For this review, take the finished solid that the model builds, in its own axes (mm). A direction names the side the tool comes from. Coordinates: 2 decimals unless noted, no trailing zeros. Loops run counter-clockwise (first coordinate to the right, second up) from the corner with the lowest first, then second, coordinate; pieces in that order, holes last. Notation, with made-up numbers: M 5.5,-11 L 10.5,-11 A15 ccw 10.5,-5 Z; hole C 89,80 d9. An arc over 180 degrees is marked long. Use one line per item in the form item = value.
```python
from build123d import *

# Parameters (mm, degrees)
SKETCH1_W           = 47
SKETCH1_H           = 55.5
BOSS_EXTRUDE1_DEPTH = 15
CUT_EXTRUDE4_DEPTH  = 54
FILLET1_R           = 7
FILLET2_R           = 7
SKETCH3_W           = 4.401923789
SKETCH3_H           = 6.5
CUT_EXTRUDE5_DEPTH  = 54
SKETCH4_W           = 1
SKETCH4_H           = 1
CUT_EXTRUDE6_DEPTH  = 54
CUT_EXTRUDE7_DEPTH  = 20
CUT_EXTRUDE8_DEPTH  = 5
BOSS_EXTRUDE3_DEPTH = 1.5
CUT_EXTRUDE9_DEPTH  = 57


with BuildPart() as part:
    # Sketch1 → Boss-Extrude1 (new body)
    with BuildSketch(Plane(origin=(0, 0, 0), x_dir=(1, 0, 0), z_dir=(0, 1, 0))):
        with Locations((23.5, -27.75)):
            Rectangle(SKETCH1_W, SKETCH1_H)
    extrude(amount=BOSS_EXTRUDE1_DEPTH)

    # Sketch2 → Cut-Extrude4 (cut)
    with BuildSketch(Plane.XY.offset(55.5)):
        with BuildLine():
            ThreePointArc((11.098076211, 15), (8.5, 15.5), (5.901923789, 15))
            Line((5.901923789, 15), (11.098076211, 15))
        make_face()
        with BuildLine():
            Line((11.098076211, 15), (5.901923789, 15))
            ThreePointArc((5.901923789, 15), (4.574858823, 2.70403013), (15.5, 8.5))
            ThreePointArc((15.5, 8.5), (14.29596987, 12.425141177), (11.098076211, 15))
        make_face()
        with BuildLine():
            ThreePointArc((26.098076211, 15), (23.5, 15.5), (20.901923789, 15))
            Line((20.901923789, 15), (26.098076211, 15))
        make_face()
        with BuildLine():
            Line((26.098076211, 15), (20.901923789, 15))
            ThreePointArc((20.901923789, 15), (19.574858823, 2.70403013), (30.5, 8.5))
            ThreePointArc((30.5, 8.5), (29.29596987, 12.425141177), (26.098076211, 15))
        make_face()
        with BuildLine():
            ThreePointArc((45.5, 8.5), (44.29596987, 12.425141177), (41.098076211, 15))
            Line((41.098076211, 15), (35.901923789, 15))
            ThreePointArc((35.901923789, 15), (34.574858823, 2.70403013), (45.5, 8.5))
        make_face()
        with BuildLine():
            Line((35.901923789, 15), (41.098076211, 15))
            ThreePointArc((41.098076211, 15), (38.5, 15.5), (35.901923789, 15))
        make_face()
    extrude(amount=-CUT_EXTRUDE4_DEPTH, mode=Mode.SUBTRACT)

    # Fillet1
    fillet1_edges = [part.edges().sort_by_distance(p)[0] for p in [
        (47, 15, 27.75),
    ]]
    fillet(fillet1_edges, radius=FILLET1_R)

    # Fillet2
    fillet2_edges = [part.edges().sort_by_distance(p)[0] for p in [
        (0, 15, 27.75),
    ]]
    fillet(fillet2_edges, radius=FILLET2_R)

    # Sketch3 → Cut-Extrude5 (cut)
    with BuildSketch(Plane.XY.offset(55.5)):
        with Locations((28.299038106, 11.75)):
            Rectangle(SKETCH3_W, SKETCH3_H)
        with Locations((33.700961895, 11.75)):
            Rectangle(SKETCH3_W, SKETCH3_H)
        with Locations((13.299038106, 11.75)):
            Rectangle(SKETCH3_W, SKETCH3_H)
        with Locations((18.700961895, 11.75)):
            Rectangle(SKETCH3_W, SKETCH3_H)
    extrude(amount=-CUT_EXTRUDE5_DEPTH, mode=Mode.SUBTRACT)

    # Sketch4 → Cut-Extrude6 (cut)
    with BuildSketch(Plane.XY.offset(55.5)):
        with Locations((16, 14.5)):
            Rectangle(SKETCH4_W, SKETCH4_H)
        with Locations((31, 14.5)):
            Rectangle(SKETCH4_W, SKETCH4_H)
    extrude(amount=-CUT_EXTRUDE6_DEPTH, mode=Mode.SUBTRACT)

    # Sketch5 → Cut-Extrude7 (cut)
    with BuildSketch(Plane.ZY.offset(-15.5)):
        Polygon((6.5, 14), (50.5, 14), (40.5, 7), (16.5, 7), align=None)
    extrude(amount=-CUT_EXTRUDE7_DEPTH, mode=Mode.SUBTRACT)

    # Sketch5_2 → Cut-Extrude8 (cut)
    with BuildSketch(Plane.ZY.offset(-15.5)):
        Polygon((6.5, 14), (50.5, 14), (40.5, 7), (16.5, 7), align=None)
    extrude(amount=CUT_EXTRUDE8_DEPTH, mode=Mode.SUBTRACT)

    # Sketch6 → Boss-Extrude3 (add)
    with BuildSketch(Plane.XY.offset(55.5)):
        with BuildLine():
            Line((0, 0), (47, 0))
            Line((47, 0), (47, 8))
            ThreePointArc((47, 8), (44.949747468, 12.949747468), (40, 15))
            Line((40, 15), (7, 15))
            ThreePointArc((7, 15), (2.050252532, 12.949747468), (0, 8))
            Line((0, 8), (0, 0))
        make_face()
    extrude(amount=BOSS_EXTRUDE3_DEPTH)

    # Sketch7 → Cut-Extrude9 (cut)
    with BuildSketch(Plane.XY.offset(57)):
        Polygon((16, 8), (16, 15), (47, 15), (47, 0), (16, 0), align=None)
    extrude(amount=-CUT_EXTRUDE9_DEPTH, mode=Mode.SUBTRACT)

    # Mirror1: part across plane


with BuildPart() as part_1:
    add(part.part)
    add(part.part.mirror(Plane(origin=(16, 8, 0), x_dir=(0, 0, 1), z_dir=(-1, 0, 0))))


solid = part_1.part
```
1. Consider section B-B on y = 12.25. Write out the cut boundary in (x, z).
Computed values:
outline = M 1.44,0 L 30.56,0 L 30.56,57 L 1.44,57 Z; hole M 2.59,1.5 L 15.5,1.5 L 15.5,9 L 16.5,9 L 16.5,1.5 L 29.41,1.5 L 29.41,55.5 L 16.5,55.5 L 16.5,48 L 15.5,48 L 15.5,55.5 L 2.59,55.5 Z
2. Tool access review of faces 4 (the face through (16, 15, 1)), 5 (the face through (27.44, 2.714, 28.878)), 6 (the face through (15.5, 11, 51)): name each direction out of +Z, -Z, +X, -X, +Y, -Y from which nothing blocks a thin tool from reaching the whole face with its end or side.
Computed values:
face_4 = +Z, -Z, +X, -X, +Y
face_5 = none
face_6 = +Y
3. Consider section C-C on z = 46. Write out the cut boundary in (x, y).
Computed values:
outline = M 0,0 L 32,0 L 32,8 A7 ccw 26.45,14.85 A7 cw long 16.5,8.5 L 16.5,10.85 L 15.5,10.85 L 15.5,8.5 A7 cw long 5.55,14.85 A7 ccw 0,8 Z
4. Consider section A-A on x = 8.5. Write out the cut boundary in (y, z).
Computed values:
outline = M 0,0 L 15,0 L 15,1.5 L 1.5,1.5 L 1.5,55.5 L 15,55.5 L 15,57 L 0,57 Z
5. Draft analysis for pull direction Y (two halves, no side actions). For faces 1 (the face through (4.56, 2.714, 28.878)), 2 (the face through (0, 4, 28)), 3 (the face through (16, 15, 56)), state which applies: +Y half, -Y half, draft (parallel to the pull), parting line (faces both ways), or undercut.
Computed values:
face_1 = undercut
face_2 = draft
face_3 = +Y half
6. Consider section D-D on x = 28.5. Write out the cut boundary in (y, z).
Computed values:
outline = M 0,0 L 14.06,0 L 14.06,57 L 0,57 Z; hole M 3.6,1.5 L 13.4,1.5 L 13.4,55.5 L 3.6,55.5 Z
7. Wall thickness on line 1 along Z through (x, y) = (22.5, 2.5); line 2 along X through (y, z) = (5.25, 39); line 3 along X through (y, z) = (3, 50.5): over which ranges is each line inside the solid? List them lowest first. Write a range as from..to.
Computed values:
line_1 = 0..1.5, 55.5..57
line_2 = 0..2.3, 14.7..17.3, 29.7..32
line_3 = 0..4.17, 12.83..19.17, 27.83..32
8. For pin 1 Ø3 at (y, z) = (11, 5.5) entering from -X; pin 2 Ø1.5 at (x, z) = (16, 26.5) entering from +Y; pin 3 Ø4 at (x, z) = (21.5, 35.5) entering from +Y, all flat-tipped, find the tip position at first contact; note any pin that passes through.
Computed values:
pin_1 = 0.16
pin_2 = 7
pin_3 = 2.76
